from build123d import *

# Parameters (mm, degrees)
F0_W     = 50.8
F0_H     = 19.05
F2_W     = 16.002
F2_H     = 34.798
F4_R     = 3.048
F6_DEPTH = 19.051


with BuildPart() as f1:
    # F0 (on Front) → F1 (revolve)
    with BuildSketch(Plane.XZ):
        with Locations((-44.45, 9.525)):
            Rectangle(F0_W, F0_H)
    revolve(axis=Axis((0, 0, 39.3560769007), (0, 0, 1)))

    # F2 (on Front) → F3 (revolve)
    with BuildSketch(Plane.XZ):
        with Locations((-27.051, 36.449)):
            Rectangle(F2_W, F2_H)
    revolve(axis=Axis((0, 0, 39.3560769007), (0, 0, 1)))

    # F4
    f4_edges = [f1.edges().sort_by_distance(p)[0] for p in [
        (35.052, 0, 53.848),
        (69.85, 0, 19.05),
        (35.052, 0, 19.05),
    ]]
    fillet(f4_edges, radius=F4_R)

    # F5 (on face) → F6 (cut, through all)
    with BuildSketch(Plane.XY.offset(19.05)):
        with BuildLine():
            ThreePointArc((-6.3389523479, 53.4735896226), (0, 47.498), (6.3389523479, 53.4735896226))
            ThreePointArc((6.3389523479, 53.4735896226), (0, 53.848), (-6.3389523479, 53.4735896226))
        make_face()
        with BuildLine():
            ThreePointArc((-6.3389523479, 53.4735896226), (0, 53.848), (6.3389523479, 53.4735896226))
            ThreePointArc((6.3389523479, 53.4735896226), (6.3472374861, 53.6607133338), (6.35, 53.848))
            ThreePointArc((6.35, 53.848), (-0.1872866662, 60.1952374861), (-6.3389523479, 53.4735896226))
        make_face()
        with BuildLine():
            ThreePointArc((-47.498, 0), (-49.2273936601, 4.3557429965), (-53.4735896226, 6.3389523479))
            ThreePointArc((-53.4735896226, 6.3389523479), (-53.848, 0), (-53.4735896226, -6.3389523479))
            ThreePointArc((-53.4735896226, -6.3389523479), (-49.2273936601, -4.3557429965), (-47.498, 0))
        make_face()
        with BuildLine():
            ThreePointArc((-53.4735896226, -6.3389523479), (-53.848, 0), (-53.4735896226, 6.3389523479))
            ThreePointArc((-53.4735896226, 6.3389523479), (-60.198, 0), (-53.4735896226, -6.3389523479))
        make_face()
        with BuildLine():
            ThreePointArc((53.4735896226, 6.3389523479), (53.7543159104, 3.175), (53.848, 0))
            ThreePointArc((53.848, 0), (53.7543159104, -3.175), (53.4735896226, -6.3389523479))
            ThreePointArc((53.4735896226, -6.3389523479), (58.2037429965, -4.6206063399), (60.198, 0))
            ThreePointArc((60.198, 0), (58.2037429965, 4.6206063399), (53.4735896226, 6.3389523479))
        make_face()
        with BuildLine():
            ThreePointArc((53.4735896226, -6.3389523479), (53.7543159104, -3.175), (53.848, 0))
            ThreePointArc((53.848, 0), (53.7543159104, 3.175), (53.4735896226, 6.3389523479))
            ThreePointArc((53.4735896226, 6.3389523479), (47.498, 0), (53.4735896226, -6.3389523479))
        make_face()
        with BuildLine():
            ThreePointArc((-6.3389523479, -53.4735896226), (0, -53.848), (6.3389523479, -53.4735896226))
            ThreePointArc((6.3389523479, -53.4735896226), (0, -47.498), (-6.3389523479, -53.4735896226))
        make_face()
        with BuildLine():
            ThreePointArc((6.35, -53.848), (6.3472374861, -53.6607133338), (6.3389523479, -53.4735896226))
            ThreePointArc((6.3389523479, -53.4735896226), (0, -53.848), (-6.3389523479, -53.4735896226))
            ThreePointArc((-6.3389523479, -53.4735896226), (-0.1872866662, -60.1952374861), (6.35, -53.848))
        make_face()
    extrude(amount=-F6_DEPTH, mode=Mode.SUBTRACT)


solid = f1.part
Verification items for the finished model (mm, model axes). A direction names the side the tool comes from. Give positions to 0.01 mm unless a question says otherwise; leave off trailing zeros. Loops run counter-clockwise (first coordinate to the right, second up) from the corner with the lowest first, then second, coordinate; pieces in that order, holes last.
1) Thickness scan on line 1 along Y through (x, z) = (0, 27); line 2 along Y through (x, z) = (5, 7). Record the ranges inside material, lowest first.
2) Depth check by flat-ended pin: pin 1 Ø10 at (x, z) = (20, 39) entering from -Y; pin 2 Ø2 at (x, z) = (29.5, 11.5) entering from -Y; pin 3 Ø2 at (x, z) = (-3, 9) entering from +Y; pin 4 Ø1.5 at (x, y) = (-7.5, -16.5) entering from +Z. Enter the tip coordinate at first touch or a pass-through.
3) Sectioned sample at B-B, the plane z = 46.5. Enter the section's corners in (x, y), then the cut area to 3 significant figures.
4) Sectioned sample at A-A, the plane x = 0. Enter the section's corners in (y, z).
5) Set-up check for faces 1 (the flat face through (-29, 29, 19.05)), 2 (the flat face through (-15, 15, 0)): record each of +Z, -Z, +X, -X, +Y, -Y from which the full face is reachable in a straight line by a thin tool's end or side.
6) Draft check along Y on faces 3 (the cylindrical face through (55.431, 42.503, 8.113)), 4 (the cylindrical face through (15.12, 11.59, 27.3)), 5 (the flat face through (-14, 14, 53.848)). Enter one of: pulls with the +Y half, pulls with the -Y half, needs draft (parallel to the pull), parting line crosses it, or undercut.
Answers:
1. line 1: y = -35.05 to -19.05, 19.05 to 35.05
1. line 2: y = -69.67 to -57.76, -49.93 to -18.38, 18.38 to 49.93, 57.76 to 69.67
2. pin 1: stops at y = -31.68
2. pin 2: stops at y = -63.77
2. pin 3: stops at y = 69.82
2. pin 4: passes through
3. outline: circle Ø70.1 at (0, 0); hole circle Ø38.1 at (0, 0)
3. area: 2,720 mm2
4. outline: (-69.85, 0) - (-60.2, 0) - (-60.2, 19.05) - (-66.8, 19.05) arc R3.05 ccw to (-69.85, 16) - close; (-47.5, 0) - (-19.05, 0) - (-19.05, 53.85) - (-32, 53.85) arc R3.05 ccw to (-35.05, 50.8) - (-35.05, 22.1) arc R3.05 cw to (-38.1, 19.05) - (-47.5, 19.05) - close; (19.05, 0) - (47.5, 0) - (47.5, 19.05) - (38.1, 19.05) arc R3.05 cw to (35.05, 22.1) - (35.05, 50.8) arc R3.05 ccw to (32, 53.85) - (19.05, 53.85) - close; (60.2, 0) - (69.85, 0) - (69.85, 16) arc R3.05 ccw to (66.8, 19.05) - (60.2, 19.05) - close
5. face 1: +Z
5. face 2: -Z, +X, -X, +Y, -Y
6. face 3: parting line crosses it
6. face 4: undercut
6. face 5: needs draft
